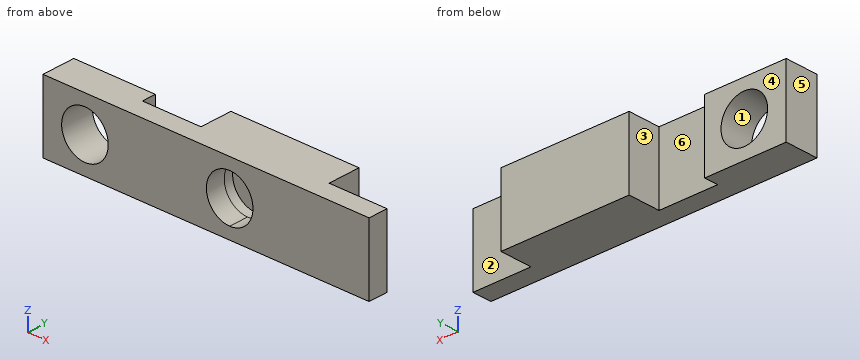
```python
from build123d import *

# Parameters (mm, degrees)
SKETCH1_W               = 140
SKETCH1_H               = 30
BOSS_EXTRUDE1_DEPTH     = 8.3
SKETCH3_W               = 35
SKETCH3_H               = 30
BOSS_EXTRUDE2_DEPTH     = 6
CUT_EXTRUDE1_DEPTH      = 6
CUT_EXTRUDE1_DEPTH_BACK = 8.3
SKETCH2_R               = 10
SKETCH4_W               = 55
SKETCH4_H               = 30
BOSS_EXTRUDE3_DEPTH     = 3.89
SKETCH5_R               = 10
CUT_EXTRUDE2_DEPTH      = 144.890548682
SKETCH7_W               = 55
SKETCH7_H               = 30
BOSS_EXTRUDE4_DEPTH     = 10


with BuildPart() as part:
    # Sketch1 → Boss-Extrude1 (new body)
    with BuildSketch(Plane(origin=(0, 0, 0), x_dir=(1, 0, 0), z_dir=(0, 1, 0))):
        with Locations((70, 15)):
            Rectangle(SKETCH1_W, SKETCH1_H)
    extrude(amount=BOSS_EXTRUDE1_DEPTH)

    # Sketch3 → Boss-Extrude2 (add)
    with BuildSketch(Plane(origin=(0, 8.3, 0), x_dir=(1, 0, 0), z_dir=(0, 1, 0))):
        with Locations((17.5, 15)):
            Rectangle(SKETCH3_W, SKETCH3_H)
    extrude(amount=BOSS_EXTRUDE2_DEPTH)

    # Sketch2 → Cut-Extrude1 (cut, two sides: drawn at the far end of the back side and taken through both)
    with BuildSketch(Plane(origin=(0, 8.3, 0), x_dir=(1, 0, 0), z_dir=(0, 1, 0)).offset(-CUT_EXTRUDE1_DEPTH_BACK)):
        with Locations(Location((18, 15, 0), (0, 0, 270))):
            Circle(SKETCH2_R)
        with Locations(Location((80.14, 15, 0), (0, 0, 90))):
            Circle(SKETCH2_R)
    extrude(amount=CUT_EXTRUDE1_DEPTH + CUT_EXTRUDE1_DEPTH_BACK, mode=Mode.SUBTRACT)

    # Sketch4 → Boss-Extrude3 (add)
    with BuildSketch(Plane(origin=(0, 8.3, 0), x_dir=(1, 0, 0), z_dir=(0, 1, 0))):
        with Locations((87.64, 15)):
            Rectangle(SKETCH4_W, SKETCH4_H)
    extrude(amount=BOSS_EXTRUDE3_DEPTH)

    # Sketch5 → Cut-Extrude2 (cut, through all)
    with BuildSketch(Plane.XZ):
        with Locations(Location((80.14, -15, 0), (0, 0, 90))):
            Circle(SKETCH5_R)
    extrude(amount=-CUT_EXTRUDE2_DEPTH, mode=Mode.SUBTRACT)

    # Sketch7 → Boss-Extrude4 (add)
    with BuildSketch(Plane(origin=(0, 12.19, 0), x_dir=(1, 0, 0), z_dir=(0, 1, 0))):
        with Locations((87.64, 15)):
            Rectangle(SKETCH7_W, SKETCH7_H)
    extrude(amount=BOSS_EXTRUDE4_DEPTH)


solid = part.part
```
CAD build for the part. Positions are in the model's coordinates, mm. Face numbers are marked on the shaded views. A direction names the side the tool comes from. Give positions to 0.01 mm unless a question says otherwise; leave off trailing zeros. Order: outer loops, then holes, each group sorted by start corner. A loop starts at its lowest first (then second) coordinate and runs counter-clockwise, first axis right, second up. Notation, with made-up numbers: M -22.5,51 L -13.5,51 A13 ccw -13.5,74 Z; hole C -0.5,-26 d9. An arc over 180 degrees is marked long. Put each result on its own line as item: value. Start each with the question number.
(1) Saw through at B-B, the plane x = 18. Write the cut outline in (y, z), then the cut area to 3 significant figures.
(2) Saw through at D-D, the plane z = -21. Write the cut outline in (x, y), then the cut area to 3 significant figures.
(3) Saw through at A-A, the plane y = 9.5. Write the cut outline in (x, z), then the cut area to 3 significant figures.
(4) Drill centre lines: line 1 along X through (y, z) = (7.5, -15); line 2 along Z through (x, y) = (80.14, 10.7); line 3 along X through (y, z) = (8.5, -28.5). Where is each one in solid material? Low to high.
(5) Mould opens along X. For the marked faces 4, 5 and 6 say: +X half, -X half, draft (parallel to the pull), parting line (faces both ways), or undercut.
(6) Flat gauge pins, fed straight in: pin 1 Ø4 at (y, z) = (16.5, -22.5) entering from -X; pin 2 Ø1.5 at (y, z) = (11, -21.5) entering from -X; pin 3 Ø1.5 at (x, z) = (25.5, -5) entering from +Y; pin 4 Ø6 at (x, z) = (79, -17.5) entering from -Y. Where does each tip first touch, or does it go through?
(7) Which spindle directions (+Z, -Z, +X, -X, +Y, -Y) get a long thin tool onto all of the face, cutting with end or side? Do the marked faces 1, 2 and 3. Say none if no direction does.
(8) Saw through at C-C, the plane z = -15. Write the cut outline in (x, y).
Check result:
1. outline: M 0,-30 L 14.3,-30 L 14.3,-25 L 0,-25 Z; M 0,-5 L 14.3,-5 L 14.3,0 L 0,0 Z
1. area: 143 mm2
2. outline: M 0,0 L 10,0 L 10,14.3 L 0,14.3 Z; M 26,0 L 72.14,0 L 72.14,12.19 L 88.14,12.19 L 88.14,0 L 140,0 L 140,8.3 L 115.14,8.3 L 115.14,22.19 L 60.14,22.19 L 60.14,8.3 L 35,8.3 L 35,14.3 L 26,14.3 Z
2. area: 1,710 mm2
3. outline: M 0,-30 L 35,-30 L 35,0 L 0,0 Z; M 60.14,-30 L 115.14,-30 L 115.14,0 L 60.14,0 Z; hole C 18,-15 d20; hole C 80.14,-15 d20
3. area: 2,070 mm2
4. line 1: x = 0 to 8, 28 to 70.14, 90.14 to 140
4. line 2: z = -30 to -25, -5 to 0
4. line 3: x = 0 to 35, 60.14 to 115.14
5. face 4: draft
5. face 5: -X half
5. face 6: undercut
6. pin 1: stops at x = 60.14
6. pin 2: stops at x = 0
6. pin 3: stops at y = 14.3
6. pin 4: stops at y = 12.19
7. face 1: +Y, -Y
7. face 2: +Z, -Z, +X, +Y
7. face 3: +Z, -Z, +Y
8. outline: M 0,0 L 8,0 L 8,14.3 L 0,14.3 Z; M 28,0 L 70.14,0 L 70.14,12.19 L 90.14,12.19 L 90.14,0 L 140,0 L 140,8.3 L 115.14,8.3 L 115.14,22.19 L 60.14,22.19 L 60.14,8.3 L 35,8.3 L 35,14.3 L 28,14.3 Z
